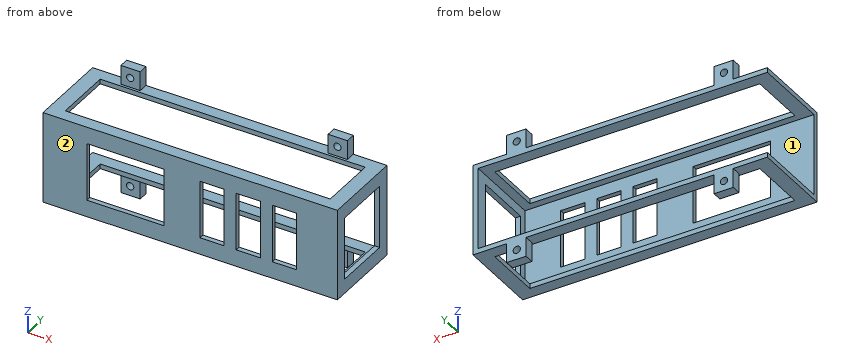
from build123d import *

# Parameters (mm, degrees)
SKETCH1_R              = 1.5
BOSS_EXTRUDE2_DEPTH    = 34
SKETCH3_W              = 120
SKETCH3_H              = 34
CUT_EXTRUDE1_DEPTH     = 32
CUT_EXTRUDE4_START     = -8
CUT_EXTRUDE4_OUTLINE_W = 8
CUT_EXTRUDE4_OUTLINE_H = 30
CUT_EXTRUDE4_DEPTH     = 8
CUT_EXTRUDE5_DEPTH     = 8
SKETCH8_W              = 8
SKETCH8_H              = 30
CUT_EXTRUDE6_DEPTH     = 8
SKETCH9_W              = 8
SKETCH9_H              = 30
CUT_EXTRUDE7_DEPTH     = 8
SKETCH10_W             = 110
SKETCH10_H             = 24
CUT_EXTRUDE8_DEPTH     = 2
SKETCH11_W             = 110
SKETCH11_H             = 24
CUT_EXTRUDE9_DEPTH     = 2
SKETCH12_W             = 26
SKETCH12_H             = 24
CUT_EXTRUDE11_DEPTH    = 2.17
SKETCH13_W             = 10
SKETCH13_H             = 24
SKETCH13_W_2           = 32
CUT_EXTRUDE12_DEPTH    = 2


# Read off the part's stored shape, not the designer's step: Cut-Extrude4
with BuildPart() as part:
    # Sketch1 → Boss-Extrude2 (new body)
    with BuildSketch(Plane(origin=(0, 0, 0), x_dir=(1, 0, 0), z_dir=(0, 1, 0))):
        Polygon((0, 0), (14.166139068, 0), (14.166139068, -8), (22.166139068, -8), (22.166139068, 0), (100.166139068, 0), (100.166139068, -8), (108.166139068, -8), (108.166139068, 0), (122.166139068, 0), (122.166139068, 38), (108.166139068, 38), (108.166139068, 46), (100.166139068, 46), (100.166139068, 38), (22.166139068, 38), (22.166139068, 46), (14.166139068, 46), (14.166139068, 38), (0, 38), align=None)
        with Locations(Location((18, 42, 0), (0, 0, 270))):
            Circle(SKETCH1_R, mode=Mode.SUBTRACT)
        with Locations(Location((18, -4, 0), (0, 0, 270))):
            Circle(SKETCH1_R, mode=Mode.SUBTRACT)
        with Locations(Location((104, -4, 0), (0, 0, 90))):
            Circle(SKETCH1_R, mode=Mode.SUBTRACT)
        with Locations(Location((104, 42, 0), (0, 0, 90))):
            Circle(SKETCH1_R, mode=Mode.SUBTRACT)
    extrude(amount=BOSS_EXTRUDE2_DEPTH)

    # Sketch3 → Cut-Extrude1 (cut)
    with BuildSketch(Plane(origin=(0, 34, 0), x_dir=(1, 0, 0), z_dir=(0, 1, 0))):
        with Locations((60, 19)):
            Rectangle(SKETCH3_W, SKETCH3_H)
    extrude(amount=-CUT_EXTRUDE1_DEPTH, mode=Mode.SUBTRACT)

    # Cut-Extrude4 outline → Cut-Extrude4 (cut)
    with BuildSketch(Plane.ZY.offset(-14.166139068).offset(CUT_EXTRUDE4_START)):
        with Locations((4, 15)):
            Rectangle(CUT_EXTRUDE4_OUTLINE_W, CUT_EXTRUDE4_OUTLINE_H)
    extrude(amount=CUT_EXTRUDE4_DEPTH, mode=Mode.SUBTRACT)

    # Sketch7 → Cut-Extrude5 (cut)
    with BuildSketch(Plane(origin=(108.166139068, 0, 0), x_dir=(0, 0, -1), z_dir=(1, 0, 0))):
        Polygon((-4, 30), (0, 30), (0, 0), (-8, 0), (-8, 30), align=None)
    extrude(amount=-CUT_EXTRUDE5_DEPTH, mode=Mode.SUBTRACT)

    # Sketch8 → Cut-Extrude6 (cut)
    with BuildSketch(Plane(origin=(108.166139068, 0, 0), x_dir=(0, 0, -1), z_dir=(1, 0, 0))):
        with Locations((42, 15)):
            Rectangle(SKETCH8_W, SKETCH8_H)
    extrude(amount=-CUT_EXTRUDE6_DEPTH, mode=Mode.SUBTRACT)

    # Sketch9 → Cut-Extrude7 (cut)
    with BuildSketch(Plane.ZY.offset(-14.166139068)):
        with Locations((-42, 15)):
            Rectangle(SKETCH9_W, SKETCH9_H)
    extrude(amount=-CUT_EXTRUDE7_DEPTH, mode=Mode.SUBTRACT)

    # Sketch10 → Cut-Extrude8 (cut)
    with BuildSketch(Plane(origin=(0, 0, -38), x_dir=(-1, 0, 0), z_dir=(0, 0, -1))):
        with Locations((-61.166139068, 17)):
            Rectangle(SKETCH10_W, SKETCH10_H)
    extrude(amount=-CUT_EXTRUDE8_DEPTH, mode=Mode.SUBTRACT)

    # Sketch11 → Cut-Extrude9 (cut)
    with BuildSketch(Plane.XY):
        with Locations((61.166139068, 17)):
            Rectangle(SKETCH11_W, SKETCH11_H)
    extrude(amount=-CUT_EXTRUDE9_DEPTH, mode=Mode.SUBTRACT)

    # Sketch12 → Cut-Extrude11 (cut)
    with BuildSketch(Plane(origin=(122.166139068, 0, 0), x_dir=(0, 0, -1), z_dir=(1, 0, 0))):
        with Locations((19, 17)):
            Rectangle(SKETCH12_W, SKETCH12_H)
    extrude(amount=-CUT_EXTRUDE11_DEPTH, mode=Mode.SUBTRACT)

    # Sketch13 → Cut-Extrude12 (cut)
    with BuildSketch(Plane.XZ):
        with Locations((100.166139068, -19)):
            Rectangle(SKETCH13_W, SKETCH13_H)
        with Locations((85.166139068, -19)):
            Rectangle(SKETCH13_W, SKETCH13_H)
        with Locations((70.166139068, -19)):
            Rectangle(SKETCH13_W, SKETCH13_H)
        with Locations((34.16188968, -19)):
            Rectangle(SKETCH13_W_2, SKETCH13_H)
    extrude(amount=-CUT_EXTRUDE12_DEPTH, mode=Mode.SUBTRACT)


solid = part.part
Here's how the part is built. I have some questions about the finished solid (model axes, mm). Face numbers are marked on the shaded views. Coordinates: 2 decimals unless noted, no trailing zeros. Order: outer loops, then holes, each group sorted by start corner. A loop starts at its lowest first (then second) coordinate and runs counter-clockwise, first axis right, second up. Notation, with made-up numbers: M 63.25,-11 L 74.25,-11 A9 cw 74.25,5 Z; hole C 4.5,73 d6. An arc over 180 degrees is marked long. Answer as CSV lines item,"result".
Item 1: Imagine slicing it at D-D on x = 104. Give the number of separate pieces and of enclosed holes in the cut face, plus the area to 3 significant figures.
Results found:
separate pieces,"6"
enclosed holes,"0"
area,"100 mm2"
Item 2: Imagine slicing it at B-B on y = 25. Write out the boundary of the cut face in (x, z), plus the area to 3 significant figures.
Results found:
outline,"M 0,-38 L 6.17,-38 L 6.17,-36 L 0,-36 Z; M 0,-2 L 6.17,-2 L 6.17,0 L 0,0 Z; M 116.17,-38 L 122.17,-38 L 122.17,-32 L 120,-32 L 120,-36 L 116.17,-36 Z; M 116.17,-2 L 120,-2 L 120,-6 L 122.17,-6 L 122.17,0 L 116.17,0 Z"
area,"66.0 mm2"
Item 3: If I drill on line 1 (Z direction, x = 18, y = 30.85); line 2 (X direction, y = 31, z = 4); line 3 (Z direction, x = 56, y = 2.5), over which ranges is the centre line in solid material (lowest first)?
Results found:
line 1,"-46 to -43.5, -40.5 to -36, -2 to 2.5, 5.5 to 8"
line 2,"14.17 to 16.5, 19.5 to 22.17, 100.17 to 102.5, 105.5 to 108.17"
line 3,"-38 to -36, -2 to 0"
Item 4: Imagine slicing it at C-C on z = 4. Write out the boundary of the cut face in (x, y), plus the area to 3 significant figures.
Results found:
outline,"M 14.17,30 L 16.5,30 L 16.5,34 L 14.17,34 Z; M 19.5,30 L 22.17,30 L 22.17,34 L 19.5,34 Z; M 100.17,30 L 102.5,30 L 102.5,34 L 100.17,34 Z; M 105.5,30 L 108.17,30 L 108.17,34 L 105.5,34 Z"
area,"40.0 mm2"
Item 5: For pin 1 (4 mm diameter, centred on x = 104, z = 4, fed in from -Y); pin 2 (16 mm diameter, centred on x = 85, y = 14, fed in from +Z); pin 3 (1.5 mm diameter, centred on x = 79, z = -6, fed in from +Y); pin 4 (2 mm diameter, centred on x = 87, y = 1.5, fed in from -Z), each with a flat end and sliding along its axis, tell me the tip position at first contact or that it passes through.
Results found:
pin 1,"y = 30"
pin 2,"through"
pin 3,"y = 2"
pin 4,"z = -38"
Item 6: We'd pull the mould along Z, two halves only. Please class the marked faces 1 and 2: +Z half, -Z half, draft (parallel to the pull), parting line (faces both ways), or undercut.
Results found:
face 1,"undercut"
face 2,"draft"
Item 7: Imagine slicing it at A-A on x = 60. Write out the boundary of the cut face in (y, z), plus the area to 3 significant figures.
Results found:
outline,"M 0,-38 L 5,-38 L 5,-36 L 2,-36 L 2,-2 L 5,-2 L 5,0 L 0,0 Z; M 29,-38 L 34,-38 L 34,-36 L 29,-36 Z; M 29,-2 L 34,-2 L 34,0 L 29,0 Z"
area,"108 mm2"
